Autodesk Inventor part; units mm, degrees
ref_plane "YZ Plane" through (0, 0, 0) normal (1, 0, 0) x (0, 1, 0)
ref_plane "XZ Plane" through (0, 0, 0) normal (0, 1, 0) x (-1, 0, 0)
ref_plane "XY Plane" through (0, 0, 0) normal (0, 0, 1) x (1, 0, 0)
sketch "Sketch1" plane through (0, 0, 0) normal (0, 0, 1) x (1, 0, 0)
  arc A0 (0, 550) -> (-200, 512.3475) centre (0, 0) ccw construction
  line L0 (-472.3938, -281.6809) -> (-252.3938, -281.6809) construction
  line L1 (-489.0365, 251.6809) -> (-252.3938, 251.6809) construction
  line L2 (-150, 323.3356) -> (-150, 512.3475) construction
  line L3 (-472.3938, 281.6809) -> (-252.3938, 281.6809) construction
  line L4 (-472.3938, -251.6809) -> (-252.3938, -251.6809) construction
  line L5 (-356.435, 15) -> (-576.435, 15) construction
  line L6 (-472.3938, -281.6809) -> (-472.3938, -251.6809) construction
  line L7 (-252.3938, -281.6809) -> (-252.3938, -251.6809) construction
  line L8 (-252.3938, 281.6809) -> (-252.3938, 251.6809) construction
  line L9 (-472.3938, 281.6809) -> (-472.3938, 251.6809) construction
  line L10 (-356.435, 15) -> (-356.435, -15) construction
  line L11 (-356.435, -15) -> (-576.435, -15) construction
  line L12 (-576.435, -15) -> (-576.435, 15) construction
  arc A1 (0, 356.435) -> (-150, 323.3356) centre (0, 0) ccw construction
  arc A2 (-150, -323.3356) -> (0, -356.435) centre (0, 0) ccw construction
  arc A3 (-256.5, -512.3475) -> (-260, -512.3475) centre (-258.25, -512.3475) ccw
  arc A4 (-290, -512.3475) -> (-293.5, -512.3475) centre (-291.75, -512.3475) ccw
  line L13 (-356.1192, -15) -> (-549.7954, -15) construction
  line L14 (-252.3938, 251.6809) -> (-489.0365, 251.6809) construction
  arc A5 (-192.6667, 512.3475) -> (-190, 512.3475) centre (-191.3333, 512.3475) ccw construction
  line L15 (-157.3333, 512.3475) -> (-150, 512.3475) construction
  line L16 (-192.6667, 512.3475) -> (-200, 512.3475) construction
  arc A6 (-160, 512.3475) -> (-157.3333, 512.3475) centre (-158.6667, 512.3475) ccw construction
  line L17 (-171.25, 517.8475) -> (-175, 517.8475) construction
  line L18 (-171.25, 520.5142) -> (-171.25, 525.1809) construction
  line L19 (-161.3333, 532.3475) -> (-188.6667, 532.3475) construction
  line L20 (-190, 531.0142) -> (-190, 512.3475) construction
  line L21 (-160, 531.0142) -> (-160, 512.3475) construction
  arc A7 (-160, 531.0142) -> (-161.3333, 532.3475) centre (-161.3333, 531.0142) ccw construction
  arc A8 (-188.6667, 532.3475) -> (-190, 531.0142) centre (-188.6667, 531.0142) ccw construction
  line L22 (-171.25, 527.8475) -> (-175, 527.8475) construction
  line L23 (-175, 532.3475) -> (-175, 535.9358) construction
  line L24 (-175, 517.8475) -> (-175, 527.8475) construction
  arc A9 (-171.25, 517.8475) -> (-171.25, 520.5142) centre (-171.25, 519.1809) ccw construction
  arc A10 (-171.25, 525.1809) -> (-171.25, 527.8475) centre (-171.25, 526.5142) ccw construction
  line L25 (-178.75, 517.8475) -> (-175, 517.8475) construction
  arc A11 (-178.75, 520.5142) -> (-178.75, 517.8475) centre (-178.75, 519.1809) ccw construction
  line L26 (-178.75, 520.5142) -> (-178.75, 525.1809) construction
  arc A12 (-178.75, 527.8475) -> (-178.75, 525.1809) centre (-178.75, 526.5142) ccw construction
  line L27 (-178.75, 527.8475) -> (-175, 527.8475) construction
  line L28 (-362.3938, -251.6809) -> (-362.3938, -293.6041)
  arc A13 (-389.2055, -291.6809) -> (-389.2055, -288.1809) centre (-389.2055, -289.9309) ccw
  line L29 (-389.2055, -291.6809) -> (-396.7055, -291.6809)
  line L30 (-396.7055, -281.6809) -> (-472.3938, -281.6809)
  line L31 (-328.082, -281.6809) -> (-252.3938, -281.6809)
  line L32 (-252.3938, -287.3475) -> (-250, -287.3475)
  arc A14 (-150, 323.3356) -> (-252.3938, -251.6809) centre (0, 0) ccw construction
  arc A15 (-200, 512.3475) -> (-472.3938, -281.6809) centre (0, 0) ccw construction
  line L33 (-300, -512.3475) -> (-300, -491.6809)
  line L34 (-260, -512.3475) -> (-260, -519.3475)
  line L35 (-290, -519.3475) -> (-290, -512.3475)
  line L36 (-256.5, -512.3475) -> (-250, -512.3475)
  line L37 (-293.5, -512.3475) -> (-300, -512.3475)
  arc A16 (-396.7055, -288.1809) -> (-396.7055, -291.6809) centre (-396.7055, -289.9309) ccw
  line L38 (-396.7055, -281.6809) -> (-396.7055, -288.1809)
  line L39 (-389.2055, -288.1809) -> (-389.2055, -274.6809)
  arc A17 (-335.582, -288.1809) -> (-335.582, -291.6809) centre (-335.582, -289.9309) ccw
  line L40 (-335.582, -291.6809) -> (-328.082, -291.6809)
  arc A18 (-328.082, -291.6809) -> (-328.082, -288.1809) centre (-328.082, -289.9309) ccw
  line L41 (-328.082, -281.6809) -> (-328.082, -288.1809)
  line L42 (-335.582, -288.1809) -> (-335.582, -274.6809)
  arc A19 (-252.3938, -283.8475) -> (-252.3938, -287.3475) centre (-252.3938, -285.5975) ccw
  line L43 (-252.3938, -283.8475) -> (-252.3938, -281.6809)
  line L44 (-335.582, -274.6809) -> (-389.2055, -274.6809)
  arc A20 (-472.3938, -281.6809) -> (-313.5, -451.9046) centre (0, 0) ccw
  line L45 (-250, -512.3475) -> (-250, -287.3475)
  line L46 (-300, -491.6809) -> (-300, -451.9046)
  arc A21 (-300, -451.9046) -> (-303.5, -451.9046) centre (-301.75, -451.9046) ccw
  line L47 (-313.5, -451.9046) -> (-303.5, -451.9046)
  line L48 (-290, -519.3475) -> (-260, -519.3475)
  point P0 (0, 512.3475)
  point P1 (0, -512.3475)
  point P2 (-59.9119, -534.1417)
  point P3 (-160, 532.3475)
  point P4 (-190, 532.3475)
  point P5 (-335.582, -268.123)
  point P6 (-389.2055, -268.123)
  dimension "d13" = 550
  dimension "d17" = 200
  dimension "d18" = 0
  dimension "d54" = 220
  dimension "d56" = 220
  dimension "d57" = 30
  dimension "d59" = 30
  dimension "d62" = 252.3938
  dimension "d73" = 236.6809
  dimension "d74" = 236.6809
  dimension "d75" = 576.435
  dimension "d76" = 472.3938
  dimension "d77" = 472.3938
  dimension "d78" = 30
  dimension "d81" = 220
  dimension "d82" = 252.3938
  dimension "d85" = 356.435
  dimension "d88" = 3.5
  dimension "d91" = 3.5
  dimension "d105" = 2.6667
  dimension "d106" = 30
  dimension "d107" = 20
  dimension "d108" = 2.6667
  dimension "d109" = 1.3333
  dimension "d110" = 7.3333
  dimension "d111" = 7.3333
  dimension "d112" = 7.5
  dimension "d113" = 3.75
  dimension "d114" = 3.75
  dimension "d140" = 7.5
  dimension "d171" = 1.75
  dimension "d172" = 10
  dimension "d173" = 3.5
  dimension "d176" = 7
  dimension "d179" = 230.6667
  dimension "d182" = 3.5
  dimension "d183" = 7
extrude "Extrusion1" add sketch "Sketch1" along normal blind 7
properties part number "Support A1 - V2"
Build history of the part. All positions in model axes, mm. A direction names the side the tool comes from. Give positions to 0.01 mm unless a question says otherwise; leave off trailing zeros. Loops run counter-clockwise (first coordinate to the right, second up) from the corner with the lowest first, then second, coordinate; pieces in that order, holes last. Notation, with made-up numbers: (47.25, 25.25) - (84.25, 25.25) arc R25 cw to (84.25, 54.25) - close; hole circle Ø9 at (28.5, -25.5). An arc over 180 degrees is marked (long way). Write item = value, one per line. Start each with the question number.
1) Band-saw the part on C-C on y = -490. Give the cut face in (x, z), plus the area to 3 significant figures.
2) Tool access for faces 1 (the flat face through (-309, -451.905, 3)), 2 (the flat face through (-335.582, -282, 3)), 3 (the flat face through (-253, -512.347, 3)), 4 (the flat face through (-434, -281.681, 3)): list every direction of +Z, -Z, +X, -X, +Y, -Y with a clear straight run to the whole face (end or side of a thin tool).
3) Probe probe 1 along X at (y, z) = (-493, 6.5); probe 2 along Y at (x, z) = (-264.5, 2.25); probe 3 along Y at (x, z) = (-316, 6.75). List the from-to ranges inside material, lowest first. Write a range as from..to.
4) Band-saw the part on B-B on x = -286. Give the cut face in (y, z), plus the area to 3 significant figures.
5) Band-saw the part on A-A on z = 3.5. Give the cut face in (x, y).
6) Drop flat-ended pins along their axis: pin 1 Ø2 at (x, z) = (-347.5, 2) entering from -Y; pin 2 Ø1 at (y, z) = (-474, 3.5) entering from -X; pin 3 Ø1.7 at (y, z) = (-283, 3) entering from +X; pin 4 Ø2 at (x, y) = (-364, -340) entering from -Z. Give the stop position or say it passes through.
7) Pull direction X, two halves, no side cores. Call faces 5 (the flat face through (-332, -291.681, 3)), 6 (the flat face through (-300, -483, 3)), 7 (the flat face through (-260, -516, 3)), 8 (the flat face through (-275, -519.347, 3)): +X half, -X half, draft (parallel to the pull), parting line (faces both ways), or undercut.
Final values:
q1.outline = (-300, 0) - (-250, 0) - (-250, 7) - (-300, 7) - close
q1.area = 350 mm²
q2.face_1 = +Z, -Z, -X, -Y
q2.face_2 = +Z, -Z, +Y
q2.face_3 = +Z, -Z, +X, -Y
q2.face_4 = +Z, -Z, -X, +Y
q3.probe_1 = -300..-250
q3.probe_2 = -519.35..-281.68
q3.probe_3 = -450.16..-281.68
q4.outline = (-519.35, 0) - (-281.68, 0) - (-281.68, 7) - (-519.35, 7) - close
q4.area = 1,660 mm²
q5.outline = (-472.39, -281.68) arc R550 ccw to (-313.5, -451.9) - (-303.5, -451.9) arc R1.75 cw to (-300, -451.9) - (-300, -512.35) - (-293.5, -512.35) arc R1.75 cw to (-290, -512.35) - (-290, -519.35) - (-260, -519.35) - (-260, -512.35) arc R1.75 cw to (-256.5, -512.35) - (-250, -512.35) - (-250, -287.35) - (-252.39, -287.35) arc R1.75 cw to (-252.39, -283.85) - (-252.39, -281.68) - (-328.08, -281.68) - (-328.08, -288.18) arc R1.75 cw to (-328.08, -291.68) - (-335.58, -291.68) arc R1.75 cw to (-335.58, -288.18) - (-335.58, -274.68) - (-389.21, -274.68) - (-389.21, -288.18) arc R1.75 cw to (-389.21, -291.68) - (-396.71, -291.68) arc R1.75 cw to (-396.71, -288.18) - (-396.71, -281.68) - close
q6.pin_1 = -427.13
q6.pin_2 = -300
q6.pin_3 = -252.39
q6.pin_4 = 0
q7.face_5 = undercut
q7.face_6 = -X half
q7.face_7 = +X half
q7.face_8 = draft
